Could you check a few things on this model? Use its own coordinates, in mm. Round coordinates to 2 decimals unless told otherwise and drop trailing zeros. Write each loop counter-clockwise with the first axis right and the second up, starting at its lowest first coordinate (ties: lowest second). Pieces come first, ordered by that corner, then holes. Notation, with made-up numbers: (-18.75, -40) -> (35.25, -40) arc R36 cw to (35.25, -3) -> close; hole circle Ø11 at (75.25, -23). An arc over 180 degrees is marked (long way). Return JSON: item names as keys, results as strings.
Autodesk Inventor part; units mm, degrees
ref_plane "YZ Plane" through (0, 0, 0) normal (1, 0, 0) x (0, 1, 0)
ref_plane "XZ Plane" through (0, 0, 0) normal (0, 1, 0) x (-1, 0, 0)
ref_plane "XY Plane" through (0, 0, 0) normal (0, 0, 1) x (1, 0, 0)
sketch "Sketch1" plane through (0, 0, 0) normal (0, 1, 0) x (-1, 0, 0)
  line L0 (55, 175) -> (-55, 175)
  line L1 (-55, 175) -> (-55, -175)
  line L2 (-55, -175) -> (55, -175)
  line L3 (55, -175) -> (55, 175)
  line L4 (55, 175) -> (-55, -175) construction
  line L5 (-55, 175) -> (55, -175) construction
  point P0 (0, 0)
  dimension "d0" = 110
  dimension "d1" = 350
extrude "Extrusion1" add sketch "Sketch1" along normal blind 3
sketch "Sketch2" plane through (0, 3, 0) normal (0, 1, 0) x (1, 0, 0)
  circle A0 centre (-47.5, 145) radius 2.5
  circle A1 centre (-32.5, 145) radius 2.5
  circle A2 centre (-47.5, 130) radius 2.5
  circle A3 centre (-32.5, 130) radius 2.5
  circle A4 centre (47.5, 145) radius 2.5
  circle A5 centre (32.5, 145) radius 2.5
  circle A6 centre (32.5, 130) radius 2.5
  circle A7 centre (47.5, 130) radius 2.5
  circle A8 centre (-47.5, -145) radius 2.5
  circle A9 centre (-32.5, -145) radius 2.5
  circle A10 centre (-47.5, -130) radius 2.5
  circle A11 centre (-32.5, -130) radius 2.5
  circle A12 centre (47.5, -130) radius 2.5
  circle A13 centre (32.5, -130) radius 2.5
  circle A14 centre (32.5, -145) radius 2.5
  circle A15 centre (47.5, -145) radius 2.5
  point P0 (0, 0)
  dimension "d4" = 5
  dimension "d5" = 5
  dimension "d6" = 5
  dimension "d7" = 5
  dimension "d8" = 5
  dimension "d9" = 5
  dimension "d10" = 5
  dimension "d11" = 5
  dimension "d12" = 5
  dimension "d13" = 5
  dimension "d14" = 5
  dimension "d15" = 5
  dimension "d16" = 5
  dimension "d17" = 5
extrude "Extrusion2" cut sketch "Sketch2" against normal blind 77.9625
sketch "Sketch3" plane through (0, 3, 0) normal (0, 1, 0) x (1, 0, 0)
  circle A0 centre (0, -165) radius 3
  point P0 (0, 0)
  dimension "d20" = 6
extrude "Extrusion3" cut sketch "Sketch3" against normal blind 75.725
sketch "Sketch4" plane through (0, 3, 0) normal (0, 1, 0) x (1, 0, 0)
  circle A0 centre (-40.0264, 38.7331) radius 1.375
  circle A1 centre (45.9736, 38.7331) radius 1.375
  circle A2 centre (45.9736, -19.2669) radius 1.375
  circle A3 centre (-40.0264, -19.2669) radius 1.375
  line L0 (-50.0264, -35.6669) -> (-50.0264, 42.1331)
  line L1 (-49.4264, 42.7331) -> (49.3736, 42.7331)
  line L2 (49.9736, 42.1331) -> (49.9736, -35.6669)
  line L3 (39.4736, -37.5169) -> (48.4736, -37.5169)
  line L4 (49.3736, -36.2669) -> (-49.4264, -36.2669)
  circle A4 centre (-40.0264, 46.7331) radius 1.375
  circle A5 centre (45.9736, 46.7331) radius 1.375
  circle A6 centre (45.9736, 104.7331) radius 1.375
  circle A7 centre (-40.0264, 104.7331) radius 1.375
  line L5 (-50.0264, 121.1331) -> (-50.0264, 43.3331)
  line L6 (49.9736, 43.3331) -> (49.9736, 121.1331)
  line L7 (39.4736, 122.9831) -> (48.4736, 122.9831)
  line L8 (49.3736, 121.7331) -> (-49.4264, 121.7331)
  point P0 (0, 0)
  point P1 (0, 85.4662)
extrude "Extrusion4" cut sketch "Sketch4" against normal blind 476.725 contours A4 | A5 | A6 | A7
sketch "Sketch7" plane through (0, 0, 0) normal (0, -1, 0) x (1, 0, 0)
  circle A0 centre (30.058, 56.5394) radius 1.5
  circle A1 centre (30.058, 116.5394) radius 1.5
  circle A2 centre (-29.942, 56.5394) radius 1.5
  circle A3 centre (-29.942, 116.5394) radius 1.5
  circle A4 centre (21.6655, 65.4546) radius 1.319
  circle A5 centre (21.6655, 108.4546) radius 1.319
  circle A6 centre (-21.3345, 65.4546) radius 1.319
  circle A7 centre (-21.3345, 108.4546) radius 1.319
  line L0 (35.058, 51.5394) -> (35.058, 121.5394)
  line L1 (35.058, 121.5394) -> (-34.942, 121.5394)
  line L2 (-34.942, 121.5394) -> (-34.942, 51.5394)
  line L3 (-34.942, 51.5394) -> (35.058, 51.5394)
  point P0 (0, 0)
extrude "Extrusion6" cut sketch "Sketch7" against normal blind 157.6375 contours A0 | A1 | A2 | A3
sketch "Sketch8" plane through (0, 0, 0) normal (0, -1, 0) x (1, 0, 0)
  circle A0 centre (-6.448, -35.5938) radius 2
  circle A1 centre (-6.4424, -28.5958) radius 2
  circle A2 centre (-48.518, -35.5603) radius 2
  circle A3 centre (-48.5124, -28.5623) radius 2
  circle A4 centre (-48.5025, -16.1623) radius 2
  circle A5 centre (-48.4797, 12.4797) radius 2
  circle A6 centre (-6.4097, 12.4462) radius 2
  line L0 (-51.4396, 18.8876) -> (-3.4396, 18.8494)
  line L1 (-51.485, -38.1124) -> (-51.4396, 18.8876)
  line L2 (-3.4396, 18.8494) -> (-3.485, -38.1506)
  line L3 (-3.485, -38.1506) -> (-51.485, -38.1124)
  circle A7 centre (48.5726, -35.5524) radius 2
  circle A8 centre (48.5782, -28.5544) radius 2
  circle A9 centre (6.5026, -35.5189) radius 2
  circle A10 centre (6.5082, -28.5209) radius 2
  circle A11 centre (6.5181, -16.1209) radius 2
  circle A12 centre (6.5409, 12.5211) radius 2
  circle A13 centre (48.6109, 12.4876) radius 2
  line L4 (3.581, 18.929) -> (51.581, 18.8908)
  line L5 (3.5356, -38.071) -> (3.581, 18.929)
  line L6 (51.581, 18.8908) -> (51.5356, -38.1092)
  line L7 (51.5356, -38.1092) -> (3.5356, -38.071)
  point P0 (0, 0)
  point P1 (0.4743, -5.9122)
extrude "Extrusion7" cut sketch "Sketch8" against normal blind 73.5 contours A0 | A2 | A5 | A6 | A7 | A9 | A12 | A13
sketch "Sketch9" plane through (0, 3, 0) normal (0, 1, 0) x (1, 0, 0)
  line L0 (30, -45) -> (50, -45)
  line L1 (50, -45) -> (50, -25)
  line L2 (50, -25) -> (30, -25)
  line L3 (30, -25) -> (30, -45)
  line L4 (30, -45) -> (50, -25) construction
  line L5 (50, -45) -> (30, -25) construction
  line L6 (-50, -45) -> (-30, -45)
  line L7 (-30, -45) -> (-30, -25)
  line L8 (-30, -25) -> (-50, -25)
  line L9 (-50, -25) -> (-50, -45)
  line L10 (-50, -45) -> (-30, -25) construction
  line L11 (-30, -45) -> (-50, -25) construction
  point P0 (0, 0)
  point P1 (40, -35)
  point P2 (-40, -35)
  dimension "d31" = 20
  dimension "d32" = 20
  dimension "d33" = 20
extrude "Extrusion8" cut sketch "Sketch9" against normal blind 163.0375
sketch "Sketch10" plane through (0, 3, 0) normal (0, 1, 0) x (1, 0, 0)
  line L0 (40, 159) -> (-40, 159)
  line L1 (-40, 159) -> (-40, 171)
  line L2 (-40, 171) -> (40, 171)
  line L3 (40, 171) -> (40, 159)
  line L4 (40, 159) -> (-40, 171) construction
  line L5 (-40, 159) -> (40, 171) construction
  point P0 (0, 0)
  point P1 (0, 165)
  dimension "d36" = 80
  dimension "d37" = 12
extrude "Extrusion9" cut sketch "Sketch10" against normal blind 159.225
sketch "Sketch11" plane through (0, 3, 0) normal (0, 1, 0) x (1, 0, 0)
  line L0 (10, -122.5215) -> (-10, -122.5215)
  line L1 (-10, -122.5215) -> (-10, -77.5215)
  line L2 (-10, -77.5215) -> (10, -77.5215)
  line L3 (10, -77.5215) -> (10, -122.5215)
  line L4 (10, -122.5215) -> (-10, -77.5215) construction
  line L5 (-10, -122.5215) -> (10, -77.5215) construction
  point P0 (0, 0)
  point P1 (0, -100.0215)
  dimension "d40" = 20
  dimension "d41" = 45
extrude "Extrusion10" cut sketch "Sketch11" against normal blind 113.825
properties part number "plat" material "Nylon 6/6"
1) I want a section at A-A, the plane x = 0. Please give me the cut outline in (y, z), and give its area (3 significant figures).
Return value:
{"outline": "(0, -175) -> (3, -175) -> (3, -171) -> (0, -171) -> close; (0, -159) -> (3, -159) -> (3, 77.52) -> (0, 77.52) -> close; (0, 122.52) -> (3, 122.52) -> (3, 162) -> (0, 162) -> close; (0, 168) -> (3, 168) -> (3, 175) -> (0, 175) -> close", "area": "861 mm²"}
2) Thinking about a two-plate mould opening in Z: for faces 1 (the face through (1, 0, 2)), 2 (the face through (1.61, 1.52, 162.47)), which applies, pulls with the +Z half, pulls with the -Z half, needs draft (parallel to the pull), parting line crosses it, or undercut?
Return value:
{"face 1": "needs draft", "face 2": "undercut"}
3) I want a section at D-D, the plane z = 30.5. Please give me the cut outline in (x, y).
Return value:
{"outline": "(-55, 0) -> (-50, 0) -> (-50, 3) -> (-55, 3) -> close; (-30, 0) -> (30, 0) -> (30, 3) -> (-30, 3) -> close; (50, 0) -> (55, 0) -> (55, 3) -> (50, 3) -> close"}
4) Will this pin go through, and if not, where does the flat tip stop? pin 1 Ø4.5 at (x, z) = (47.5, -130) entering from -Y.
Return value:
{"pin 1": "through"}
5) If I drill on probe 1 along X at (y, z) = (1.6, -145); probe 2 along Z at (x, y) = (7, 0.75); probe 3 along Z at (x, y) = (-37.5, 0.85), over which ranges is the centre line in solid material (lowest first)? Write a range as [from, to].
Return value:
{"probe 1": "[-55, -50], [-45, -35], [-30, 30], [35, 45], [50, 55]", "probe 2": "[-175, -171], [-159, -37.46], [-33.58, 10.57], [14.47, 77.52], [122.52, 175]", "probe 3": "[-175, -171], [-159, 25], [45, 175]"}
6) I want a section at C-C, the plane x = -18. Please give me the cut outline in (y, z).
Return value:
{"outline": "(0, -175) -> (3, -175) -> (3, -171) -> (0, -171) -> close; (0, -159) -> (3, -159) -> (3, 175) -> (0, 175) -> close"}
7) I want a section at B-B, the plane z = 165. Please give me the cut outline in (x, y).
Return value:
{"outline": "(-55, 0) -> (-3, 0) -> (-3, 3) -> (-55, 3) -> close; (3, 0) -> (55, 0) -> (55, 3) -> (3, 3) -> close"}
